from build123d import *

# Parameters (mm, degrees)
SKETCH1_W           = 6.5
SKETCH1_H           = 5
BOSS_EXTRUDE1_DEPTH = 0.75
SKETCH2_R           = 1.1
CUT_EXTRUDE1_DEPTH  = 5.168333


with BuildPart() as part:
    # Sketch1 → Boss-Extrude1 (new body)
    with BuildSketch(Plane(origin=(0, 0, 0), x_dir=(1, 0, 0), z_dir=(0, 1, 0))):
        Rectangle(SKETCH1_W, SKETCH1_H)
    extrude(amount=BOSS_EXTRUDE1_DEPTH)

    # Sketch2 → Cut-Extrude1 (cut, through all)
    with BuildSketch(Plane(origin=(0, 0, 0), x_dir=(1, 0, 0), z_dir=(0, 1, 0))):
        with Locations(Location((0, 0.484711092, 0), (0, 0, 270))):
            Circle(SKETCH2_R)
    extrude(amount=CUT_EXTRUDE1_DEPTH, mode=Mode.SUBTRACT)


solid = part.part
Source: CAD feature listing. Evaluate the final solid. Frame: model axes, mm. Round coordinates to 2 decimals unless told otherwise and drop trailing zeros. Order: outer loops, then holes, each group sorted by start corner. A loop starts at its lowest first (then second) coordinate and runs counter-clockwise, first axis right, second up. Notation, with made-up numbers: (57.25, -32.75) - (62.25, -32.75) arc R16 cw to (62.25, -23.75) - close; hole circle Ø8 at (22, 19.5). An arc over 180 degrees is marked (long way). Use a Markdown table: item, result. Add a question column.
1. Section query A-A (x = 0). Return the cut outline in (y, z).
2. Section query C-C (y = 0.45). Return the cut outline in (x, z).
3. Mould query, pull axis X, two halves, no side actions, for faces 1 (the flat face through (-1, 0.75, 1)), 2 (the cylindrical face through (0.33, 0.37, 0.564)). Classes: +X half, -X half, draft (parallel to the pull), parting line (faces both ways), or undercut.
4. First-contact query: pin 1 (1.5 mm diameter, centred on x = 1, z = 1, fed in from -Y). Flat tip, straight axial feed; report the tip coordinate or a pass-through.
5. Line query: probe 1 along X at (y, z) = (0.5, -0.45); probe 2 along Z at (x, y) = (0, 0.5); probe 3 along X at (y, z) = (0.25, -1.25). Output: solid intervals per line, ascending.
6. Section query B-B (z = -0.8). Return the cut outline in (x, y), then the cut area to 3 significant figures.
Derived:
| question | item | result |
|---|---|---|
| 1 | outline | (0, -2.5) - (0.75, -2.5) - (0.75, -1.58) - (0, -1.58) - close; (0, 0.62) - (0.75, 0.62) - (0.75, 2.5) - (0, 2.5) - close |
| 2 | outline | (-3.25, -2.5) - (3.25, -2.5) - (3.25, 2.5) - (-3.25, 2.5) - close; hole circle Ø2.2 at (0, -0.48) |
| 3 | face 1 | draft |
| 3 | face 2 | undercut |
| 4 | pin 1 | y = 0 |
| 5 | probe 1 | -3.25 to -1.1, 1.1 to 3.25 |
| 5 | probe 2 | -2.5 to -1.58, 0.62 to 2.5 |
| 5 | probe 3 | -3.25 to -0.79, 0.79 to 3.25 |
| 6 | outline | (-3.25, 0) - (-1.05, 0) - (-1.05, 0.75) - (-3.25, 0.75) - close; (1.05, 0) - (3.25, 0) - (3.25, 0.75) - (1.05, 0.75) - close |
| 6 | area | 3.29 mm2 |
